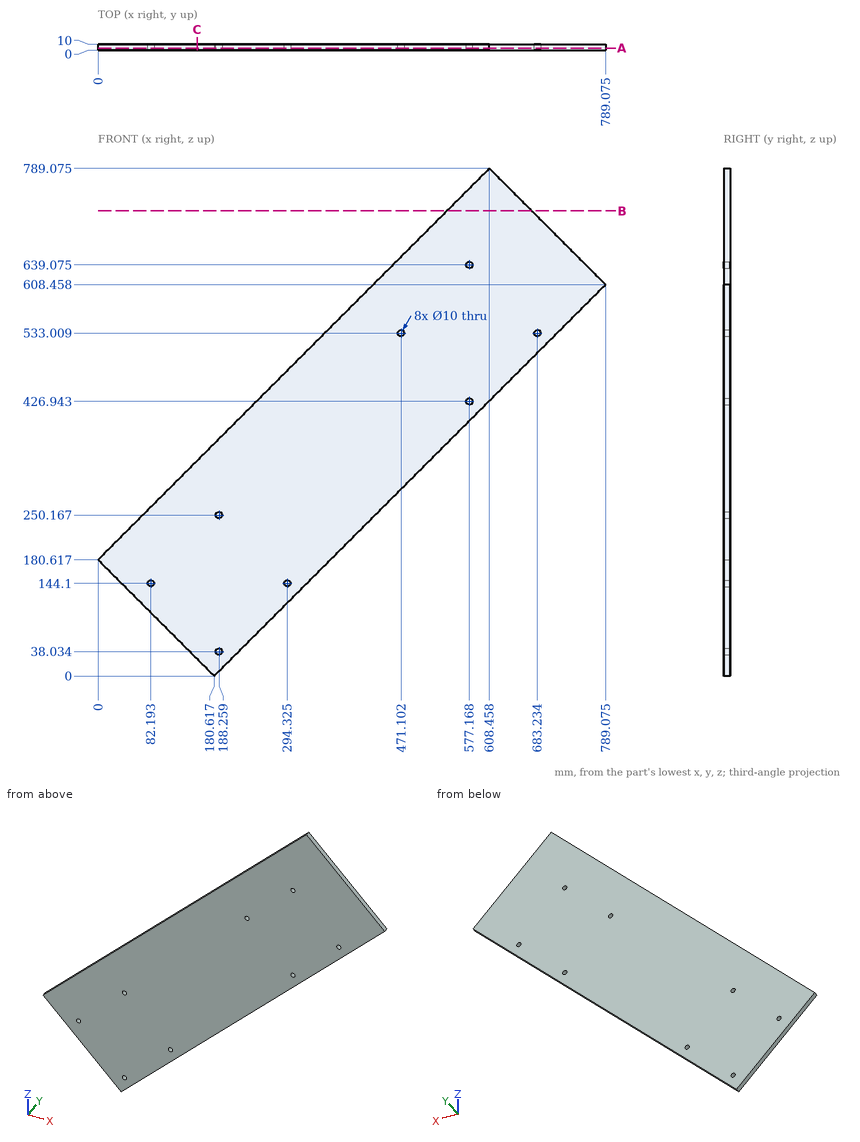
Input: dimensioned drawing with shaded views. Units: mm. Origin: part minimum x, y, z. Give positions to 0.01 mm unless a question says otherwise; leave off trailing zeros. Order: outer loops, then holes, each group sorted by start corner. A loop starts at its lowest first (then second) coordinate and runs counter-clockwise, first axis right, second up. Notation, with made-up numbers: (-22, -35) -> (23, -35) arc R15 cw to (23, -29) -> close; hole circle Ø5 at (-7, 17.5). An arc over 180 degrees is marked (long way). Use one line per item in the form item = value.
1) Line query: probe 1 along Z at (x, y) = (48, 4.75) (1 decimal); probe 2 along X at (y, z) = (7, 455) (1 decimal); probe 3 along X at (y, z) = (6.75, 345.5) (1 decimal). Output: solid intervals per line, ascending.
Response values:
probe_1 = 132.6 to 228.6
probe_2 = 274.4 to 635.6
probe_3 = 164.9 to 526.1
2) First-contact query: pin 1 Ø3 at (y, z) = (8, 269.5) entering from -X (1 decimal); pin 2 Ø2 at (y, z) = (7.5, 357.5) entering from +X (1 decimal); pin 3 Ø1.5 at (y, z) = (2.5, 428.5) entering from -X (1 decimal); pin 4 Ø6 at (x, z) = (188.26, 38.03) entering from -Y. Flat tips, straight axial feed; report the tip coordinate or a pass-through.
Response values:
pin_1 = 87.4
pin_2 = 539.1
pin_3 = 247.1
pin_4 = through
3) Section A-A, the plane y = 3.75. Count the separate pieces of the cut face and the enclosed holes in it, and give its area (3 significant figures).
Response values:
separate_pieces = 1
enclosed_holes = 8
area = 219,000 mm^2
4) Section B-B, the plane z = 723. Return loops of the section in (x, y).
Response values:
outline = (542.38, 0) -> (674.53, 0) -> (674.53, 10) -> (542.38, 10) -> close
5) Section C-C, the plane x = 154. Return loops of the section in (y, z).
Response values:
outline = (0, 26.62) -> (10, 26.62) -> (10, 334.62) -> (0, 334.62) -> close
